Build history of the part. All positions in model axes, mm. Face numbers are marked on the shaded views. A direction names the side the tool comes from. Give positions to 0.01 mm unless a question says otherwise; leave off trailing zeros. Order: outer loops, then holes, each group sorted by start corner. A loop starts at its lowest first (then second) coordinate and runs counter-clockwise, first axis right, second up. Notation, with made-up numbers: (-38, 88) - (12, 88) arc R15 cw to (12, 112) - close; hole circle Ø8 at (21, 26.5). An arc over 180 degrees is marked (long way). Use a Markdown table: item, result.
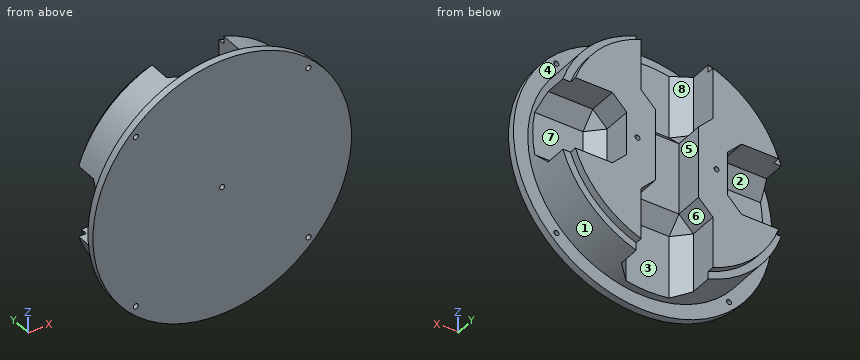
from build123d import *

# Parameters (mm, degrees)
SKETCH1_R                           = 80
BOSS_EXTRUDE1_DEPTH                 = 30
SKETCH2_R                           = 90
BOSS_EXTRUDE2_DEPTH                 = 5
SKETCH6_R                           = 75
BOSS_EXTRUDE3_DEPTH                 = 5
F_3_5_3_5_DIAMETER_HOLE1_D          = 3.5
F_3_5_3_5_DIAMETER_HOLE1_DEPTH      = 10
F_3_5_3_5_DIAMETER_HOLE1_TIP        = 1.051506083
SKETCH7_W                           = 50
SKETCH7_H                           = 110
CUT_EXTRUDE1_DEPTH                  = 30
CHAMFER1_SIZE                       = 10
SKETCH8_W                           = 30
SKETCH8_H                           = 50
CUT_EXTRUDE2_DEPTH                  = 20
F_3_5_3_5_DIAMETER_HOLE2_AT_2_COUNT = 2
F_3_5_3_5_DIAMETER_HOLE2_AT_2_PITCH = 85
F_3_5_3_5_DIAMETER_HOLE2_AT_3_COUNT = 2
F_3_5_3_5_DIAMETER_HOLE2_AT_3_PITCH = 85
F_3_5_3_5_DIAMETER_HOLE2_AT_4_COUNT = 2
F_3_5_3_5_DIAMETER_HOLE2_AT_4_PITCH = 85
F_3_5_3_5_DIAMETER_HOLE2_AT_5_COUNT = 2
F_3_5_3_5_DIAMETER_HOLE2_AT_5_PITCH = 85
SKETCH11_W                          = 80
SKETCH11_H                          = 50
CUT_EXTRUDE3_DEPTH                  = 30
CHAMFER2_SIZE                       = 10


with BuildPart() as part:
    # Sketch1 → Boss-Extrude1 (new body)
    with BuildSketch(Plane(origin=(0, 0, 0), x_dir=(1, 0, 0), z_dir=(0, 1, 0))):
        with Locations(Location((0, 0, 0), (0, 0, 270))):
            Circle(SKETCH1_R)
    extrude(amount=BOSS_EXTRUDE1_DEPTH)

    # Sketch2 → Boss-Extrude2 (add)
    with BuildSketch(Plane.XZ):
        with Locations(Location((0, 0, 0), (0, 0, 270))):
            Circle(SKETCH2_R)
    extrude(amount=BOSS_EXTRUDE2_DEPTH)

    # Sketch6 → Boss-Extrude3 (add)
    with BuildSketch(Plane(origin=(0, 30, 0), x_dir=(1, 0, 0), z_dir=(0, 1, 0))):
        with Locations(Location((0, 0, 0), (0, 0, 270))):
            Circle(SKETCH6_R)
    extrude(amount=BOSS_EXTRUDE3_DEPTH)

    # Ø3.5 (3.5) Diameter Hole1
    with Locations(Plane(origin=(-12.746034072, 35, -7.868896946), x_dir=(1, 0, 0), z_dir=(0, 1, 0))):
        with Locations((-14.753965928, -7.868896946), (40.246034072, -7.868896946)):
            Hole(F_3_5_3_5_DIAMETER_HOLE1_D / 2, depth=F_3_5_3_5_DIAMETER_HOLE1_DEPTH)
            with Locations((0, 0, -(F_3_5_3_5_DIAMETER_HOLE1_DEPTH + F_3_5_3_5_DIAMETER_HOLE1_TIP / 2))):  # 118° drill point
                Cone(0, F_3_5_3_5_DIAMETER_HOLE1_D / 2, F_3_5_3_5_DIAMETER_HOLE1_TIP, mode=Mode.SUBTRACT)

    # Sketch7 → Cut-Extrude1 (cut)
    with BuildSketch(Plane(origin=(0, 35, 0), x_dir=(1, 0, 0), z_dir=(0, 1, 0))):
        with Locations((0, 80)):
            Rectangle(SKETCH7_W, SKETCH7_H)
        with Locations((0, -80)):
            Rectangle(SKETCH7_W, SKETCH7_H)
    extrude(amount=-CUT_EXTRUDE1_DEPTH, mode=Mode.SUBTRACT)

    # Chamfer1
    chamfer1_edges = [part.edges().sort_by_distance(p)[0] for p in [
        (25, 5, -50.496710384),
        (-25, 5, -50.496710384),
        (-25, 20, -25),
        (0, 5, -25),
        (25, 20, -25),
        (25, 5, 50.496710384),
        (25, 20, 25),
        (-25, 5, 50.496710384),
        (0, 5, 25),
        (-25, 20, 25),
    ]]
    chamfer(chamfer1_edges, length=CHAMFER1_SIZE)

    # Sketch8 → Cut-Extrude2 (cut)
    with BuildSketch(Plane(origin=(0, 35, 0), x_dir=(1, 0, 0), z_dir=(0, 1, 0))):
        Rectangle(SKETCH8_W, SKETCH8_H)
    extrude(amount=-CUT_EXTRUDE2_DEPTH, mode=Mode.SUBTRACT)

    # Sketch9 → Ø3.5 (3.5) Diameter Hole2 (revolve, cut)
    with BuildSketch(Plane(origin=(0, 0, 0), x_dir=(0, 0, 1), z_dir=(1, 0, 0))):
        Polygon((0, 0), (0, 11.051506083), (1.75, 10), (1.75, 0), align=None)
    f_3_5_3_5_diameter_hole2 = revolve(axis=Axis((0, 6.35, 0), (0, -1, 0)), mode=Mode.SUBTRACT)

    # Ø3.5 (3.5) Diameter Hole2 at 2: Ø3.5 (3.5) Diameter Hole2 ×2
    with Locations(*[Vector(0.7071067811865478, 0, 0.7071067811865475) * (i * F_3_5_3_5_DIAMETER_HOLE2_AT_2_PITCH) for i in range(1, F_3_5_3_5_DIAMETER_HOLE2_AT_2_COUNT)]):
        add(f_3_5_3_5_diameter_hole2, mode=Mode.SUBTRACT)

    # Ø3.5 (3.5) Diameter Hole2 at 3: Ø3.5 (3.5) Diameter Hole2 ×2
    with Locations(*[Vector(-0.7071067811865477, 0, -0.7071067811865475) * (i * F_3_5_3_5_DIAMETER_HOLE2_AT_3_PITCH) for i in range(1, F_3_5_3_5_DIAMETER_HOLE2_AT_3_COUNT)]):
        add(f_3_5_3_5_diameter_hole2, mode=Mode.SUBTRACT)

    # Ø3.5 (3.5) Diameter Hole2 at 4: Ø3.5 (3.5) Diameter Hole2 ×2
    with Locations(*[Vector(-0.7071067811865476, 0, 0.7071067811865476) * (i * F_3_5_3_5_DIAMETER_HOLE2_AT_4_PITCH) for i in range(1, F_3_5_3_5_DIAMETER_HOLE2_AT_4_COUNT)]):
        add(f_3_5_3_5_diameter_hole2, mode=Mode.SUBTRACT)

    # Ø3.5 (3.5) Diameter Hole2 at 5: Ø3.5 (3.5) Diameter Hole2 ×2
    with Locations(*[Vector(0.7071067811865476, 0, -0.7071067811865476) * (i * F_3_5_3_5_DIAMETER_HOLE2_AT_5_PITCH) for i in range(1, F_3_5_3_5_DIAMETER_HOLE2_AT_5_COUNT)]):
        add(f_3_5_3_5_diameter_hole2, mode=Mode.SUBTRACT)

    # Sketch11 → Cut-Extrude3 (cut)
    with BuildSketch(Plane(origin=(0, 35, 0), x_dir=(1, 0, 0), z_dir=(0, 1, 0))):
        with Locations((75, 0)):
            Rectangle(SKETCH11_W, SKETCH11_H)
        with Locations((-75, 0)):
            Rectangle(SKETCH11_W, SKETCH11_H)
    extrude(amount=-CUT_EXTRUDE3_DEPTH, mode=Mode.SUBTRACT)

    # Chamfer2
    chamfer2_edges = [part.edges().sort_by_distance(p)[0] for p in [
        (55.496710384, 5, -25),
        (35, 20, -25),
        (55.496710384, 5, 25),
        (35, 5, 0),
        (35, 20, 25),
        (-55.496710384, 5, -25),
        (-55.496710384, 5, 25),
        (-35, 20, 25),
        (-35, 5, 0),
        (-35, 20, -25),
    ]]
    chamfer(chamfer2_edges, length=CHAMFER2_SIZE)


solid = part.part
1) Slice it at C-C (y = 9.5). Write the cut outline in (x, z), and give its area (3 significant figures).
Computed:
| item | result |
|---|---|
| outline | (-77.59, -19.5) arc R80 ccw to (-19.5, -77.59) - (-19.5, -35) - (-15, -30.5) - (15, -30.5) - (19.5, -35) - (19.5, -77.59) arc R80 ccw to (77.59, -19.5) - (45, -19.5) - (40.5, -15) - (40.5, 15) - (45, 19.5) - (77.59, 19.5) arc R80 ccw to (19.5, 77.59) - (19.5, 35) - (15, 30.5) - (-15, 30.5) - (-19.5, 35) - (-19.5, 77.59) arc R80 ccw to (-77.59, 19.5) - (-45, 19.5) - (-40.5, 15) - (-40.5, -15) - (-45, -19.5) - close |
| area | 13,400 mm² |
2) Wall check: line 1 (X direction, y = 19, z = 0); line 2 (Y direction, x = 79, z = 37.5); line 3 (Y direction, x = 57.5, z = -53). Give the ranges that are in metal, low to high. Write a range as from..to.
Computed:
| item | result |
|---|---|
| line 1 | x = -35..-15, 15..35 |
| line 2 | y = -5..0 |
| line 3 | y = -5..30 |
3) Slice it at B-B (x = 19). Write the cut outline in (y, z).
Computed:
| item | result |
|---|---|
| outline | (-5, -87.97) - (0, -87.97) - (0, -77.71) - (9, -77.71) - (9, -35) - (15, -29) - (35, -29) - (35, 29) - (15, 29) - (9, 35) - (9, 77.71) - (0, 77.71) - (0, 87.97) - (-5, 87.97) - close |
4) Slice it at A-A (z = 10.5). Write the cut outline in (x, y), and give its area (3 significant figures).
Computed:
| item | result |
|---|---|
| outline | (-89.39, -5) - (89.39, -5) - (89.39, 0) - (79.31, 0) - (79.31, 5) - (45, 5) - (35, 15) - (35, 35) - (15, 35) - (15, 15) - (-15, 15) - (-15, 35) - (-35, 35) - (-35, 15) - (-45, 5) - (-79.31, 5) - (-79.31, 0) - (-89.39, 0) - close |
| area | 3,290 mm² |
5) Tool access for the marked faces 4, 5, 6, 7 and 8: list every direction of +Z, -Z, +X, -X, +Y, -Y with a clear straight run to the whole face (end or side of a thin tool).
Computed:
| item | result |
|---|---|
| face 4 | +Y |
| face 5 | +Z, -Z, +Y |
| face 6 | -Z, +Y |
| face 7 | +X, +Y |
| face 8 | +Z, +Y |
6) Slice it at D-D (z = -44). Write the cut outline in (x, y).
Computed:
| item | result |
|---|---|
| outline | (-78.51, -5) - (78.51, -5) - (78.51, 0) - (66.81, 0) - (66.81, 30) - (60.74, 30) - (60.74, 35) - (25, 35) - (25, 15) - (15, 5) - (-15, 5) - (-25, 15) - (-25, 35) - (-60.74, 35) - (-60.74, 30) - (-66.81, 30) - (-66.81, 0) - (-78.51, 0) - close |
7) Pin check, flat tips, straight feed: P1, Ø1, axis at x = -1, z = 0, coming from the -Y side; P2, Ø4, axis at x = 0, z = 0, coming from the +Y side; P3, Ø10, axis at x = -43.5, y = 11.5, coming from the +Z side. Stop position of each tip, or through.
Computed:
| item | result |
|---|---|
| P1 | stops at y = 0 |
| P2 | stops at y = 15 |
| P3 | stops at z = 70.13 |
8) Two-plate mould, pull along Z, no slides. Class the marked faces 1, 2 and 3: +Z half, -Z half, draft (parallel to the pull), parting line (faces both ways), or undercut.
Computed:
| item | result |
|---|---|
| face 1 | parting line |
| face 2 | undercut |
| face 3 | draft |
